```python
from build123d import *

# Parameters (mm, degrees)
F1_DEPTH = 24
F2_R     = 1.5
F2_R_2   = 5
F3_DEPTH = 25
F4_R     = 0.5


with BuildPart() as f1:
    # F0 (on Top) → F1 (new body)
    with BuildSketch(Plane.XY):
        Polygon((-15.5, 0), (0, 0), (15.5, 0), (15.5, 18.5), (28.5, 18.5), (28.5, 0), (37.5, 0), (37.5, 2), (30.5, 2), (30.5, 18.5), (37.5, 18.5), (37.5, 20.5), (13.5, 20.5), (13.5, 2), (0, 2), (-13.5, 2), (-13.5, 20.5), (-37.5, 20.5), (-37.5, 18.5), (-30.5, 18.5), (-30.5, 2), (-37.5, 2), (-37.5, 0), (-28.5, 0), (-28.5, 18.5), (-15.5, 18.5), align=None)
    extrude(amount=F1_DEPTH)

    # F2 (on face) → F3 (cut)
    with BuildSketch(Plane.XZ):
        with Locations((-33.5, 12)):
            Circle(F2_R)
        with Locations((0, 12)):
            Circle(F2_R_2)
        with Locations((33.5, 12)):
            Circle(F2_R)
    extrude(amount=-F3_DEPTH, mode=Mode.SUBTRACT)

    # F4
    f4_edges = [f1.edges().sort_by_distance(p)[0] for p in [
        (-13.5, 20.5, 12),
        (13.5, 20.5, 12),
        (15.5, 0, 12),
        (-28.5, 0, 12),
        (-15.5, 0, 12),
        (28.5, 0, 12),
        (37.5, 20.5, 12),
        (37.5, 18.5, 12),
        (37.5, 2, 12),
        (37.5, 0, 12),
        (-37.5, 20.5, 12),
        (-37.5, 18.5, 12),
        (-37.5, 2, 12),
        (-37.5, 0, 12),
        (-5, 0, 12),
        (-5, 2, 12),
    ]]
    fillet(f4_edges, radius=F4_R)


solid = f1.part
```
Design review of the part built by this model. Coordinates are the model's own, in mm. A direction names the side the tool comes from. Give positions to 0.01 mm unless a question says otherwise; leave off trailing zeros. Order: outer loops, then holes, each group sorted by start corner. A loop starts at its lowest first (then second) coordinate and runs counter-clockwise, first axis right, second up. Notation, with made-up numbers: (66.5, 5) -> (124.5, 5) arc R8 ccw to (124.5, 16) -> close; hole circle Ø2 at (29.5, -35.75). An arc over 180 degrees is marked (long way). Write each question's results on one line, items separated by ' | '. Start each with the question number.
Q1. Add section A-A on x = 33.5. Give the boundary of the cut face in (y, z).
Q2. For pin 1 (2.5 mm diameter, centred on x = 33.5, z = 12, fed in from -Y); pin 2 (5.5 mm diameter, centred on y = 13.5, z = 6.5, fed in from +X); pin 3 (5 mm diameter, centred on y = 15.5, z = 12.5, fed in from -X); pin 4 (10 mm diameter, centred on x = -0.5, z = 14, fed in from +Y), all flat-tipped, find the tip position at first contact; note any pin that passes through.
Q3. Add section C-C on x = 0. Give the boundary of the cut face in (y, z).
Q4. Add section B-B on y = 4.25. Give the boundary of the cut face in (x, z), and give its area (3 significant figures).
Q5. Add section D-D on z = 12. State how many separate pieces and enclosed holes the cut face has, and give its area (3 significant figures).
Q6. Wall thickness on L1, parallel to X at y = 8, z = 22.25; L2, parallel to Z at x = 33.5, y = 19.5; L3, parallel to Y at x = -32, z = 21.75: over which ranges is each line inside the solid? List them lowest first. Write a range as from..to.
Q7. Machinability: for faces 4 (the flat face through (-35.2, 18.5, 11.8)), 5 (the flat face through (-22, 18.5, 12)), 6 (the flat face through (30.5, 10, 12)), 7 (the flat face through (13.5, 11, 12)), which of the approach directions +Z, -Z, +X, -X, +Y, -Y give a long, thin tool a straight path to every point of the face, cutting with its end or side? Answer none if there is none.
Q8. Mouldability with a two-part tool opening along X and no side actions: class faces 1 (the flat face through (-30.5, 10, 12)), 2 (the flat face through (0, 0, 6)), 3 (the cylindrical face through (-34.7, 1, 11.1)) as +X half, -X half, draft (parallel to the pull), parting line (faces both ways), or undercut.
Found:
1) outline: (0, 0) -> (2, 0) -> (2, 10.5) -> (0, 10.5) -> close; (0, 13.5) -> (2, 13.5) -> (2, 24) -> (0, 24) -> close; (18.5, 0) -> (20.5, 0) -> (20.5, 10.5) -> (18.5, 10.5) -> close; (18.5, 13.5) -> (20.5, 13.5) -> (20.5, 24) -> (18.5, 24) -> close
2) pin 1: passes through | pin 2: stops at x = 30.5 | pin 3: stops at x = -30.5 | pin 4: stops at y = 2
3) outline: (0, 0) -> (2, 0) -> (2, 6.5) arc R0.5 ccw to (1.5, 7) -> (0.5, 7) arc R0.5 ccw to (0, 6.5) -> close; (0, 17.5) arc R0.5 ccw to (0.5, 17) -> (1.5, 17) arc R0.5 ccw to (2, 17.5) -> (2, 24) -> (0, 24) -> close
4) outline: (-30.5, 0) -> (-28.5, 0) -> (-28.5, 24) -> (-30.5, 24) -> close; (-15.5, 0) -> (-13.5, 0) -> (-13.5, 24) -> (-15.5, 24) -> close; (13.5, 0) -> (15.5, 0) -> (15.5, 24) -> (13.5, 24) -> close; (28.5, 0) -> (30.5, 0) -> (30.5, 24) -> (28.5, 24) -> close | area: 192 mm2
5) separate pieces: 6 | enclosed holes: 0 | area: 281 mm2
6) L1: x = -30.5..-28.5, -15.5..-13.5, 13.5..15.5, 28.5..30.5 | L2: z = 0..10.5, 13.5..24 | L3: y = 0..2, 18.5..20.5
7) face 4: +Z, -Z, -X | face 5: +Z, -Z, -Y | face 6: +Z, -Z, +X | face 7: +Z, -Z, +Y
8) face 1: -X half | face 2: draft | face 3: undercut
